Build history of the part. All positions in model axes, mm. A direction names the side the tool comes from. Give positions to 0.01 mm unless a question says otherwise; leave off trailing zeros. Write each loop counter-clockwise with the first axis right and the second up, starting at its lowest first coordinate (ties: lowest second). Pieces come first, ordered by that corner, then holes.
Autodesk Inventor part; units mm, degrees
ref_plane "YZ Plane" through (0, 0, 0) normal (1, 0, 0) x (0, 1, 0)
ref_plane "XZ Plane" through (0, 0, 0) normal (0, 1, 0) x (-1, 0, 0)
ref_plane "XY Plane" through (0, 0, 0) normal (0, 0, 1) x (1, 0, 0)
sketch "Sketch1" plane through (0, 0, 0) normal (0, 1, 0) x (-1, 0, 0)
  line L0 (26.2836, 34.9539) -> (-35.7164, 34.9539)
  line L1 (-35.7164, 34.9539) -> (-35.7164, -34.0461)
  line L2 (-35.7164, -34.0461) -> (26.2836, -34.0461)
  line L3 (26.2836, -34.0461) -> (26.2836, 34.9539)
  circle A0 centre (11.2836, -28.0461) radius 1.75
  circle A1 centre (11.2836, -28.0461) radius 3
  circle A2 centre (-20.7164, -28.0461) radius 1.75
  circle A3 centre (-20.7164, -28.0461) radius 3
  circle A4 centre (-20.7164, 28.9539) radius 1.75
  circle A5 centre (-20.7164, 28.9539) radius 3
  circle A6 centre (11.2836, 28.9539) radius 1.75
  circle A7 centre (11.2836, 28.9539) radius 3
  line L4 (-15.7164, 34.9539) -> (-25.7164, 34.9539)
  circle A8 centre (20.2836, 26.9539) radius 2.25
  circle A9 centre (20.2836, -26.0461) radius 2.25
  circle A10 centre (-29.7164, 26.9539) radius 2.25
  circle A11 centre (-29.7164, -26.0461) radius 2.25
  circle A12 centre (20.2836, 26.9539) radius 4.5
  circle A13 centre (20.2836, -26.0461) radius 4.5
  circle A14 centre (-29.7164, -26.0461) radius 4.5
  circle A15 centre (-29.7164, 26.9539) radius 4.5
  line L5 (18.0336, 23.0568) -> (15.7836, 26.9539)
  line L6 (15.7836, 26.9539) -> (18.0336, 30.8511)
  line L7 (18.0336, 30.8511) -> (22.5336, 30.8511)
  line L8 (22.5336, 30.8511) -> (24.7836, 26.9539)
  line L9 (24.7836, 26.9539) -> (22.5336, 23.0568)
  line L10 (22.5336, 23.0568) -> (18.0336, 23.0568)
  line L11 (18.0336, -29.9432) -> (15.7836, -26.0461)
  line L12 (15.7836, -26.0461) -> (18.0336, -22.1489)
  line L13 (18.0336, -22.1489) -> (22.5336, -22.1489)
  line L14 (22.5336, -22.1489) -> (24.7836, -26.0461)
  line L15 (24.7836, -26.0461) -> (22.5336, -29.9432)
  line L16 (22.5336, -29.9432) -> (18.0336, -29.9432)
  line L17 (-31.9664, -29.9432) -> (-34.2164, -26.0461)
  line L18 (-34.2164, -26.0461) -> (-31.9664, -22.1489)
  line L19 (-31.9664, -22.1489) -> (-27.4664, -22.1489)
  line L20 (-27.4664, -22.1489) -> (-25.2164, -26.0461)
  line L21 (-25.2164, -26.0461) -> (-27.4664, -29.9432)
  line L22 (-27.4664, -29.9432) -> (-31.9664, -29.9432)
  line L23 (-31.9664, 23.0568) -> (-34.2164, 26.9539)
  line L24 (-34.2164, 26.9539) -> (-31.9664, 30.8511)
  line L25 (-31.9664, 30.8511) -> (-27.4664, 30.8511)
  line L26 (-27.4664, 30.8511) -> (-25.2164, 26.9539)
  line L27 (-25.2164, 26.9539) -> (-27.4664, 23.0568)
  line L28 (-27.4664, 23.0568) -> (-31.9664, 23.0568)
  point P0 (0, 0)
  dimension "d45" = 9
  dimension "d46" = 9
  dimension "d47" = 9
  dimension "d48" = 9
  dimension "d0" = 69
  dimension "d1" = 62
  dimension "d2" = 3.5
  dimension "d3" = 6
  dimension "d4" = 3.5
  dimension "d5" = 6
  dimension "d6" = 3.5
  dimension "d7" = 6
  dimension "d8" = 3.5
  dimension "d9" = 6
  dimension "d10" = 15
  dimension "d11" = 15
  dimension "d12" = 15
  dimension "d13" = 15
  dimension "d14" = 6
  dimension "d15" = 6
  dimension "d16" = 6
  dimension "d17" = 6
  dimension "d32" = 4.5
  dimension "d33" = 4.5
  dimension "d34" = 4.5
  dimension "d35" = 4.5
  dimension "d36" = 8
  dimension "d37" = 8
  dimension "d38" = 8
  dimension "d39" = 8
  dimension "d40" = 6
  dimension "d41" = 6
  dimension "d42" = 6
  dimension "d43" = 6
  dimension "d44" = 53
extrude "Extrusion1" add sketch "Sketch1" against normal blind 5 contours L3 L2 L1 L0 | A1 | A3 | A5 | A7 | L8 A12 | L9 L10 L5 L6 L7 L8 | A12 L9 | L7 A12 | A12 L10 | L6 A12 | A12 L5 | L14 A13 | L15 L16 L11 L12 L13 L14 | A13 L15 | L13 A13 | A13 L16 | L12 A13 | A13 L11 | L20 A14 | L21 L22 L17 L18 L19 L20 | A14 L21 | L19 A14 | A14 L22 | L18 A14 | A14 L17 | L26 A15 | L27 L28 L23 L24 L25 L26 | A15 L27 | L25 A15 | A15 L28 | L24 A15 | A15 L23
extrude "Extrusion2" cut sketch "Sketch1" against normal blind 2 contours A1 | A3 | A5 | A7
sketch "Sketch2" plane through (0, -5, 0) normal (0, -1, 0) x (1, 0, 0)
  line L0 (27.5264, 23.0228) -> (25.2764, 26.92)
  line L1 (25.2764, 26.92) -> (27.5264, 30.8171)
  line L2 (27.5264, 30.8171) -> (32.0264, 30.8171)
  line L3 (32.0264, 30.8171) -> (34.279, 26.9154)
  line L4 (34.279, 26.9154) -> (32.0264, 23.0198)
  line L5 (32.0264, 23.0198) -> (27.5264, 23.0228)
  line L6 (27.4664, -29.9432) -> (25.2764, -26.0461)
  line L7 (25.2764, -26.0461) -> (27.5264, -22.1489)
  line L8 (27.5264, -22.1489) -> (32.0264, -22.1489)
  line L9 (32.0264, -22.1489) -> (34.2164, -26.0461)
  line L10 (34.2164, -26.0461) -> (31.9664, -29.9432)
  line L11 (31.9664, -29.9432) -> (27.4664, -29.9432)
  line L12 (-22.5336, -29.9432) -> (-24.7836, -26.0461)
  line L13 (-24.7836, -26.0461) -> (-22.5336, -22.1489)
  line L14 (-22.5336, -22.1489) -> (-18.0336, -22.1489)
  line L15 (-18.0336, -22.1489) -> (-15.7836, -26.0461)
  line L16 (-15.7836, -26.0461) -> (-18.0336, -29.9432)
  line L17 (-18.0336, -29.9432) -> (-22.5336, -29.9432)
  line L18 (-22.5336, 23.0568) -> (-24.7236, 26.9539)
  line L19 (-24.7236, 26.9539) -> (-22.4736, 30.8511)
  line L20 (-22.4736, 30.8511) -> (-17.9736, 30.8511)
  line L21 (-17.9736, 30.8511) -> (-15.7236, 26.9539)
  line L22 (-15.7236, 26.9539) -> (-17.9736, 23.0568)
  line L23 (-17.9736, 23.0568) -> (-22.5336, 23.0568)
  line L24 (-26.2836, 34.9539) -> (-26.2836, -34.0461)
  line L25 (35.7164, 34.9539) -> (-26.2836, 34.9539)
  line L26 (35.7164, -34.0461) -> (35.7164, 34.9539)
  line L27 (-26.2836, -34.0461) -> (35.7164, -34.0461)
  point P0 (0, 0)
extrude "Extrusion3" cut sketch "Sketch2" against normal blind 4 contours L0 L1 L2 L3 L4 L5 | L6 L7 L8 L9 L10 L11 | L12 L13 L14 L15 L16 L17 | L18 L19 L20 L21 L22 L23
fillet "Fillet1" radius 2 8 edges at (35.7164, -2.5, -34.0461) (35.7164, -2.5, 34.9539) (-26.2836, -2.5, 34.9539) (-26.2836, -2.5, -34.0461) (-26.2836, 0, 0.4539) (4.7164, 0, -34.0461) (4.7164, 0, 34.9539) (35.7164, 0, 0.4539)
sketch "Sketch3" plane through (0, 0, 0) normal (0, 1, 0) x (1, 0, 0)
  line L0 (23.7164, 19.0461) -> (-14.2836, 19.0461)
  line L1 (-14.2836, 19.0461) -> (-14.2836, -19.9539)
  line L2 (-14.2836, -19.9539) -> (23.7164, -19.9539)
  line L3 (23.7164, -19.9539) -> (23.7164, 19.0461)
  line L4 (35.7164, -32.9539) -> (35.7164, 32.0461)
  line L5 (-26.2836, 32.0461) -> (-26.2836, -32.9539)
  line L6 (-24.2836, -34.9539) -> (33.7164, -34.9539)
  line L7 (33.7164, 34.0461) -> (-24.2836, 34.0461)
  point P0 (0, 0)
  dimension "d68" = 12
  dimension "d69" = 12
  dimension "d70" = 15
  dimension "d71" = 15
extrude "Extrusion4" cut sketch "Sketch3" against normal through all
fillet "Fillet2" radius 2 8 edges at (4.7164, 0, -19.0461) (23.7164, 0, 0.4539) (4.7164, 0, 19.9539) (-14.2836, 0, 0.4539) (4.7164, -5, 19.9539) (-14.2836, -5, 0.4539) (4.7164, -5, -19.0461) (23.7164, -5, 0.4539)
properties part number "BatteryHolder2PBase"
(1) Saw through at A-A, the plane z = -17. List the corners of the cut face in (x, y).
(2) Probe line 1 (Z direction, x = 31.5, y = -3.8); line 2 (X direction, y = -2.8, z = -2); line 3 (Z direction, x = -20, y = -3.4). List the from-to ranges inside material, lowest first.
(3) Drop flat-ended pins along their axis: pin 1 (5.5 mm diameter, centred on x = 20.72, z = 28.95, fed in from +Y); pin 2 (7 mm diameter, centred on x = 29.72, z = -26.05, fed in from +Y); pin 3 (2 mm diameter, centred on x = 20.72, z = -28.05, fed in from +Y). Give the stop position or say it passes through.
(4) Saw through at C-C, the plane x = 20. Give the number of separate pieces and of enclosed holes in the cut face, plus the area to 3 significant figures.
(5) Mould opens along X. For faces 4 (the face through (-25.713, -3.521, -33.445)), 5 (the face through (-12.668, -0.986, 26.292)), 6 (the face through (19, -2, -29)), 7 (the face through (4, -3, 34.954)) say: +X half, -X half, draft (parallel to the pull), parting line (faces both ways), or undercut.
(6) 3-axis set-ups, long thin cutter, end or side, ignore diameter. For faces 1 (the face through (-13, -2, 28)), 2 (the face through (-16.833, -3.028, 25.033)), 3 (the face through (22.465, -3.479, 29.031)): which of +Z, -Z, +X, -X, +Y, -Y reach the whole face in a straight line?
(7) Saw through at B-B, the plane x = -1. List the corners of the cut face in (y, z), plus the area to 3 significant figures.
Computed values:
1. outline: (-26.28, -5) - (-16.28, -5) arc R2 ccw to (-14.28, -3) - (-14.28, -2) arc R2 ccw to (-16.28, 0) - (-24.28, 0) arc R2 ccw to (-26.28, -2) - close; (23.72, -3) arc R2 ccw to (25.72, -5) - (35.72, -5) - (35.72, -2) arc R2 ccw to (33.72, 0) - (25.72, 0) arc R2 ccw to (23.72, -2) - close
2. line 1: z = -34.05 to -29.94, -22.15 to 23.02, 30.82 to 34.95
2. line 2: x = -26.28 to -14.28, 23.72 to 35.72
2. line 3: z = -34.05 to -29.94, -22.15 to 23.06, 30.85 to 34.95
3. pin 1: stops at y = -2
3. pin 2: stops at y = 0
3. pin 3: passes through
4. separate pieces: 4
4. enclosed holes: 0
4. area: 102 mm2
5. face 4: -X half
5. face 5: undercut
5. face 6: undercut
5. face 7: draft
6. face 1: +Y
6. face 2: -Y
6. face 3: +Y, -Y
7. outline: (-5, -34.05) - (-2, -34.05) arc R2 ccw to (0, -32.05) - (0, -21.05) arc R2 ccw to (-2, -19.05) - (-3, -19.05) arc R2 ccw to (-5, -21.05) - close; (-5, 21.95) arc R2 ccw to (-3, 19.95) - (-2, 19.95) arc R2 ccw to (0, 21.95) - (0, 32.95) arc R2 ccw to (-2, 34.95) - (-5, 34.95) - close
7. area: 145 mm2
